from build123d import *

# Parameters (mm, degrees)
SKETCH1_W           = 6
SKETCH1_H           = 5
BOSS_EXTRUDE1_DEPTH = 6
CUT_EXTRUDE1_DEPTH  = 3.5
SKETCH3_W           = 3
SKETCH3_H           = 2
BOSS_EXTRUDE2_DEPTH = 3
CUT_EXTRUDE2_DEPTH  = 3.5


with BuildPart() as part:
    # Sketch1 → Boss-Extrude1 (new body)
    with BuildSketch(Plane(origin=(0, 0, 0), x_dir=(1, 0, 0), z_dir=(0, 1, 0))):
        Rectangle(SKETCH1_W, SKETCH1_H)
    extrude(amount=BOSS_EXTRUDE1_DEPTH)

    # Sketch2 → Cut-Extrude1 (cut)
    with BuildSketch(Plane.XY.offset(2.5)):
        Polygon((3, 6), (-3, 0), (-3, 6), align=None)
    extrude(amount=-CUT_EXTRUDE1_DEPTH, mode=Mode.SUBTRACT)

    # Sketch3 → Boss-Extrude2 (add)
    with BuildSketch(Plane(origin=(0, 6, 0), x_dir=(1, 0, 0), z_dir=(0, 1, 0))):
        with Locations((1.5, 0)):
            Rectangle(SKETCH3_W, SKETCH3_H)
    extrude(amount=-BOSS_EXTRUDE2_DEPTH)

    # Sketch4 → Cut-Extrude2 (cut)
    with BuildSketch(Plane.XY.offset(1)):
        Polygon((3, 6), (-3, 4), (-3, 6), align=None)
    extrude(amount=-CUT_EXTRUDE2_DEPTH, mode=Mode.SUBTRACT)


solid = part.part
Design review of the part built by this model. Coordinates are the model's own, in mm. A direction names the side the tool comes from. Coordinates: 2 decimals unless noted, no trailing zeros. Loops run counter-clockwise (first coordinate to the right, second up) from the corner with the lowest first, then second, coordinate; pieces in that order, holes last. Notation, with made-up numbers: M 61,7 L 113,7 A21 cw 113,37 Z; hole C 35,-26 d1. An arc over 180 degrees is marked long. Use one line per item in the form item = value.
(1) For faces 1 (the face through (3, 3, 0)), 2 (the face through (0, 4, 0)), list the 3-axis set-ups (+Z, -Z, +X, -X, +Y, -Y) from which the entire face can be reached by the end or side of a thin tool; tool diameter is ignored.
Return value:
face_1 = +Z, -Z, +X, +Y, -Y
face_2 = +Z, -X, +Y
(2) Consider section D-D (y = 1.95). Write out the cut boundary in (x, z), and give its area (3 significant figures).
Return value:
outline = M -3,-2.5 L 3,-2.5 L 3,2.5 L -1.05,2.5 L -1.05,-1 L -3,-1 Z
area = 23.2 mm2
(3) For line 1 along Z through (x, y) = (-2, 4.15); line 2 along Z through (x, y) = (2, 5.2); line 3 along Y through (x, z) = (0, 1.8), list the stretches that pass through material, from the lowest coordinate up. Write a range as from..to.
Return value:
line_1 = -2.5..-1
line_2 = -2.5..1
line_3 = 0..3
(4) Consider section A-A (y = 4.45). Write out the cut boundary in (x, z), and give its area (3 significant figures).
Return value:
outline = M -1.65,-2.5 L 3,-2.5 L 3,2.5 L 1.45,2.5 L 1.45,1 L 0,1 L 0,-1 L -1.65,-1 Z
area = 15.3 mm2
(5) Consider section C-C (x = -1.5). Write out the cut boundary in (y, z), and give its area (3 significant figures).
Return value:
outline = M 0,-2.5 L 4.5,-2.5 L 4.5,-1 L 1.5,-1 L 1.5,2.5 L 0,2.5 Z
area = 12.0 mm2
(6) Consider section B-B (z = 0.7). Write out the cut boundary in (x, y), and give its area (3 significant figures).
Return value:
outline = M -3,0 L 3,0 L 3,6 L 0,5 L 0,3 Z
area = 21.0 mm2
(7) Clearance check with flat-ended pins moving along their axes: P1, Ø3, axis at x = -0.5, y = 5, coming from the +Z side; P2, Ø0.6, axis at y = 3.5, z = 0, coming from the -X side. State where each tip first meets the part, or that it passes through.
Return value:
P1 = 1
P2 = 0
